Part model, mm, in its own coordinate system. Round coordinates to 2 decimals unless told otherwise and drop trailing zeros. Loops run counter-clockwise (first coordinate to the right, second up) from the corner with the lowest first, then second, coordinate; pieces in that order, holes last. Notation, with made-up numbers: (5.25, 28.25) - (30.25, 28.25) arc R28 cw to (30.25, 55.25) - close; hole circle Ø1 at (-17, 34). An arc over 180 degrees is marked (long way). Put each result on its own line as item: value.
from build123d import *

# Parameters (mm, degrees)
SKETCH1_R           = 1.75
BOSS_EXTRUDE1_DEPTH = 56
SKETCH2_R           = 19.5
CUT_EXTRUDE1_DEPTH  = 56


with BuildPart() as part:
    # Sketch1 → Boss-Extrude1 (new body)
    with BuildSketch(Plane.XY):
        with BuildLine():
            Line((-16, -20), (16, -20))
            ThreePointArc((16, -20), (18.828427125, -18.828427125), (20, -16))
            Line((20, -16), (20, 16))
            ThreePointArc((20, 16), (18.828427125, 18.828427125), (16, 20))
            Line((16, 20), (-16, 20))
            ThreePointArc((-16, 20), (-18.828427125, 18.828427125), (-20, 16))
            Line((-20, 16), (-20, -16))
            ThreePointArc((-20, -16), (-18.828427125, -18.828427125), (-16, -20))
        make_face()
        with Locations((16, 16)):
            Circle(SKETCH1_R, mode=Mode.SUBTRACT)
        with Locations(Location((-16, 16, 0), (0, 0, 180))):
            Circle(SKETCH1_R, mode=Mode.SUBTRACT)
        with Locations(Location((16, -16, 0), (0, 0, 180))):
            Circle(SKETCH1_R, mode=Mode.SUBTRACT)
        with Locations((-16, -16)):
            Circle(SKETCH1_R, mode=Mode.SUBTRACT)
    extrude(amount=-BOSS_EXTRUDE1_DEPTH)

    # Sketch2 → Cut-Extrude1 (cut)
    with BuildSketch(Plane.XY):
        Circle(SKETCH2_R)
    extrude(amount=-CUT_EXTRUDE1_DEPTH, mode=Mode.SUBTRACT)


solid = part.part
1. Band-saw the part on B-B (y = 7). List the corners of the cut face in (x, z), plus the area to 3 significant figures.
A:
outline: (-20, -56) - (-18.2, -56) - (-18.2, 0) - (-20, 0) - close; (18.2, -56) - (20, -56) - (20, 0) - (18.2, 0) - close
area: 202 mm²
2. Two-plate mould, pull along X, no slides. Class faces 1 (the cylindrical face through (-18.797, 18.859, -27.608)), 2 (the flat face through (-4.5, 19.4, 0)), 3 (the cylindrical face through (15.772, 17.735, -27.608)): pulls with the +X half, pulls with the -X half, needs draft (parallel to the pull), parting line crosses it, or undercut.
A:
face 1: pulls with the -X half
face 2: needs draft
face 3: undercut
3. Pin check, flat tip, straight feed: P1, Ø3, axis at x = 16, y = -16, coming from the +Z side. Stop position of the tip, or through.
A:
P1: passes through
4. Probe line 1 along Y through (x, z) = (0, -21); line 2 along X through (y, z) = (-17, -34.5); line 3 along X through (y, z) = (-17.5, -18.5). List the from-to ranges inside material, lowest first. Write a range as [from, to].
A:
line 1: y = [-20, -19.5], [19.5, 20]
line 2: x = [-19.87, -17.44], [-14.56, -9.55], [9.55, 14.56], [17.44, 19.87]
line 3: x = [-19.71, -16.9], [-15.1, -8.6], [8.6, 15.1], [16.9, 19.71]
5. Band-saw the part on C-C (z = -26.5). List the corners of the cut face in (x, y).
A:
outline: (-20, -16) arc R4 ccw to (-16, -20) - (16, -20) arc R4 ccw to (20, -16) - (20, 16) arc R4 ccw to (16, 20) - (-16, 20) arc R4 ccw to (-20, 16) - close; hole circle Ø39 at (0, 0); hole circle Ø3.5 at (-16, -16); hole circle Ø3.5 at (-16, 16); hole circle Ø3.5 at (16, -16); hole circle Ø3.5 at (16, 16)
